Model file for the job. Use its own axes, mm. Face numbers are marked on the shaded views. A direction names the side the tool comes from. Round coordinates to 2 decimals unless told otherwise and drop trailing zeros. Use one line per item in the form item = value.
from build123d import *


with BuildPart() as f1:
    # F0 (on Front) → F1 (revolve)
    with BuildSketch(Plane.XZ):
        with BuildLine():
            Line((0, -105.212546), (0, 123.387454))
            Line((0, 123.387454), (-17.287159, 123.387454))
            Line((-17.287159, 123.387454), (-17.287159, 72.718156))
            Line((-17.287159, 72.718156), (-17.287159, 66.368156))
            Line((-17.287159, 66.368156), (-30.758225, 52.89709))
            Line((-30.758225, 52.89709), (-30.758225, 46.54709))
            Line((-30.758225, 46.54709), (-17.287159, 33.076024))
            Line((-17.287159, 33.076024), (-17.287159, 26.998156))
            Line((-17.287159, 26.998156), (-30.758225, 13.52709))
            Line((-30.758225, 13.52709), (-30.758225, 7.17709))
            Line((-30.758225, 7.17709), (-17.287159, -6.293976))
            Line((-17.287159, -6.293976), (-17.287159, -12.371844))
            Line((-17.287159, -12.371844), (-30.758225, -25.84291))
            Line((-30.758225, -25.84291), (-30.758225, -32.19291))
            Line((-30.758225, -32.19291), (-17.287159, -45.663976))
            Line((-17.287159, -45.663976), (-17.287159, -51.741844))
            Line((-17.287159, -51.741844), (-30.758225, -65.21291))
            Line((-30.758225, -65.21291), (-30.758225, -71.56291))
            Line((-30.758225, -71.56291), (-17.287159, -85.033976))
            Line((-17.287159, -85.033976), (-17.287159, -91.383976))
            ThreePointArc((-17.287159, -91.383976), (-28.722438, -96.749767), (-38.1, -105.212546))
            Line((-38.1, -105.212546), (0, -105.212546))
        make_face()
    revolve(axis=Axis((0, 0, 9.087454), (0, 0, -1)))


solid = f1.part
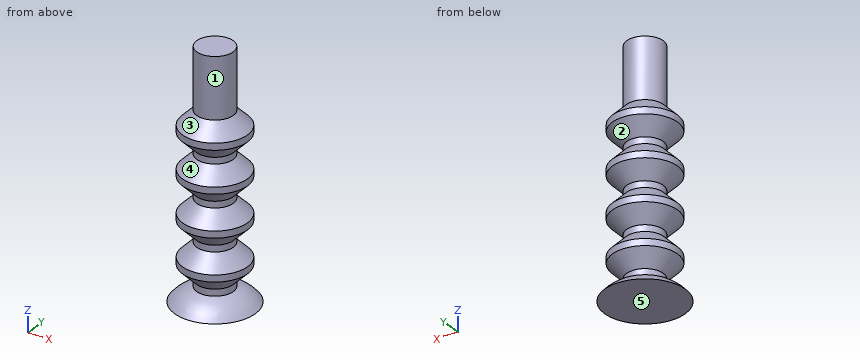
(1) Probe probe 1 along Z at (x, y) = (-24, -8); probe 2 along Z at (x, y) = (6, 29.5); probe 3 along Y at (x, z) = (-23.5, -30.5). List the from-to ranges inside material, lowest first. Write a range as [from, to].
Report:
probe_1 = [-105.21, -94.7], [-77.02, -59.75], [-37.65, -20.38], [1.72, 18.99], [41.09, 58.36]
probe_2 = [-105.21, -97.71], [-72.22, -64.56], [-32.85, -25.19], [6.52, 14.18], [45.89, 53.55]
probe_3 = [-19.84, 19.84]
(2) Slice it at A-A on y = 21. Count the separate pieces of the cut face and the enclosed holes in it, then the cut area to 3 significant figures.
Report:
separate_pieces = 5
enclosed_holes = 0
area = 3,950 mm2
(3) Pull direction Z, two halves, no side cores. Call the marked faces 1, 2 and 3: released by +Z, released by -Z, zero draft, split by the parting line, or undercut.
Report:
face_1 = zero draft
face_2 = undercut
face_3 = released by +Z
(4) Pin check, flat tips, straight feed: pin 1 (8 mm diameter, centred on y = 19.5, z = -61.5, fed in from -X); pin 2 (12 mm diameter, centred on x = 25, y = -15.5, fed in from +Z); pin 3 (12 mm diameter, centred on x = 30, z = -51, fed in from +Y); pin 4 (1.5 mm diameter, centred on y = 22, z = 51.5, fed in from -X). Stop position of each tip, or through.
Report:
pin_1 = -24.99
pin_2 = 60.24
pin_3 = through
pin_4 = -22.24
(5) Tool access for the marked faces 4 and 5: list every direction of +Z, -Z, +X, -X, +Y, -Y with a clear straight run to the whole face (end or side of a thin tool).
Report:
face_4 = none
face_5 = -Z, +X, -X, +Y, -Y
